```python
from build123d import *

# Parameters (mm, degrees)
SKETCH1_W           = 10
SKETCH1_H           = 5
BOSS_EXTRUDE1_DEPTH = 45
FILLET1_R           = 2
CUT_EXTRUDE1_DEPTH  = 10


with BuildPart() as part:
    # Sketch1 → Boss-Extrude1 (new body)
    with BuildSketch(Plane.XY):
        Rectangle(SKETCH1_W, SKETCH1_H)
    extrude(amount=BOSS_EXTRUDE1_DEPTH)

    # Fillet1
    fillet1_edges = [part.edges().sort_by_distance(p)[0] for p in [
        (-5, 0, 45),
        (0, -2.5, 45),
        (5, 0, 45),
        (0, -2.5, 0),
        (-5, 0, 0),
        (0, 2.5, 0),
        (5, 0, 0),
        (0, 2.5, 45),
        (5, -2.5, 22.5),
        (-5, -2.5, 22.5),
        (-5, 2.5, 22.5),
        (5, 2.5, 22.5),
    ]]
    fillet(fillet1_edges, radius=FILLET1_R)

    # Sketch2 → Cut-Extrude1 (cut)
    with BuildSketch(Plane.XZ.offset(2.5)):
        with BuildLine():
            Line((2.05, 42), (-2.05, 42))
            ThreePointArc((-2.05, 42), (-2.368198052, 42.131801948), (-2.5, 42.45))
            Line((-2.5, 42.45), (-2.5, 42.55))
            ThreePointArc((-2.5, 42.55), (-2.368198052, 42.868198052), (-2.05, 43))
            Line((-2.05, 43), (2.05, 43))
            ThreePointArc((2.05, 43), (2.368198052, 42.868198052), (2.5, 42.55))
            Line((2.5, 42.55), (2.5, 42.45))
            ThreePointArc((2.5, 42.45), (2.368198052, 42.131801948), (2.05, 42))
        make_face()
    extrude(amount=-CUT_EXTRUDE1_DEPTH, mode=Mode.SUBTRACT)


solid = part.part
```
Design review of the part built by this model. Coordinates are the model's own, in mm. A direction names the side the tool comes from. Coordinates: 2 decimals unless noted, no trailing zeros. Loops run counter-clockwise (first coordinate to the right, second up) from the corner with the lowest first, then second, coordinate; pieces in that order, holes last.
Q1. The part is to be moulded in two halves that separate along X. For faces 3 (the face through (0, 0, 42)), 4 (the face through (0.04, 1.93, 44.4)), 5 (the face through (4.43, 0.01, 0.6)), say which applies: +X half, -X half, draft (parallel to the pull), parting line (faces both ways), or undercut.
Reported:
face 3: undercut
face 4: draft
face 5: +X half
Q2. Tool access review of faces 1 (the face through (-5, 0, 22)), 2 (the face through (0, 0, 43)): name each direction out of +Z, -Z, +X, -X, +Y, -Y from which nothing blocks a thin tool from reaching the whole face with its end or side.
Reported:
face 1: +Z, -Z, -X, +Y, -Y
face 2: +Y, -Y
Q3. For pin 1 (2 mm diameter, centred on y = 2, z = 5.5, fed in from +X), flat-tipped, find the tip position at first contact; note if it passes through.
Reported:
pin 1: stops at x = 4.94
Q4. We need section A-A on y = -2.1. State the section outline as (x, z) points.
Reported:
outline: (-4.2, 2) arc R1.2 ccw to (-3, 0.8) - (3, 0.8) arc R1.2 ccw to (4.2, 2) - (4.2, 43) arc R1.2 ccw to (3, 44.2) - (-3, 44.2) arc R1.2 ccw to (-4.2, 43) - close; hole (-2.5, 42.45) arc R0.45 ccw to (-2.05, 42) - (2.05, 42) arc R0.45 ccw to (2.5, 42.45) - (2.5, 42.55) arc R0.45 ccw to (2.05, 43) - (-2.05, 43) arc R0.45 ccw to (-2.5, 42.55) - close
Q5. To check wall thickness, follow line 1 (Z direction, x = 0.75, y = 0.65); line 2 (Z direction, x = -1.75, y = 1.2); line 3 (Z direction, x = 2.75, y = -1.4). State the ranges of each line that lie inside material, in increasing order.
Reported:
line 1: z = 0.01 to 42, 43 to 44.99
line 2: z = 0.13 to 42, 43 to 44.87
line 3: z = 0.21 to 44.79
Q6. We need section C-C on z = 29.5. State the section outline as (x, y) points.
Reported:
outline: (-5, -0.5) arc R2 ccw to (-3, -2.5) - (3, -2.5) arc R2 ccw to (5, -0.5) - (5, 0.5) arc R2 ccw to (3, 2.5) - (-3, 2.5) arc R2 ccw to (-5, 0.5) - close
Q7. We need section D-D on x = -4.25. State the section outline as (y, z) points.
Reported:
outline: (-2.06, 2) arc R1.56 ccw to (-0.5, 0.44) - (0.5, 0.44) arc R1.56 ccw to (2.06, 2) - (2.06, 43) arc R1.56 ccw to (0.5, 44.56) - (-0.5, 44.56) arc R1.56 ccw to (-2.06, 43) - close
Q8. We need section B-B on x = 1.5. State the section outline as (y, z) points, and give its area (3 significant figures).
Reported:
outline: (-2.5, 2) arc R2 ccw to (-0.5, 0) - (0.5, 0) arc R2 ccw to (2.5, 2) - (2.5, 42) - (-2.5, 42) - close; (-2.5, 43) - (2.5, 43) arc R2 ccw to (0.5, 45) - (-0.5, 45) arc R2 ccw to start
area: 217 mm2
